Read the model definition and answer for the solid it produces. Units are mm, in the model's axes. Coordinates: 2 decimals unless noted, no trailing zeros.
Item 1: Determine the mould class of faces 1 (the face through (-276.225, 16, 0)), 2 (the face through (251, 7.27, -0.13)), 3 (the face through (-4, 16, -9.525)) for opening direction X: released by +X, released by -X, zero draft, split by the parting line, or undercut.
Item 2: Straight lines are drawn through the part: probe 1 along X at (y, z) = (21, -4.75) (3 decimals); probe 2 along X at (y, z) = (5.5, -4.75) (3 decimals); probe 3 along Y at (x, z) = (239, -6.5). For each, find the intervals that lie inside material, in ascending order.
Item 3: Each of these flat-tipped pins is pushed along its axis until it touches: P1, Ø2.5, axis at x = 225.23, y = 13.49, coming from the +Z side; P2, Ø7, axis at x = -260.55, y = 13.49, coming from the -Z side. Where does it stop, or does it pass through?
Item 4: Section A-A (z = 6.25) is taken. State how many separate pieces and enclosed holes the cut face has, then the cut area to 3 significant figures.
from build123d import *

# Parameters (mm, degrees)
SKETCH1_W                                         = 552.45
SKETCH1_H                                         = 19.05
BOSS_EXTRUDE1_DEPTH                               = 31.75
SKETCH2_R                                         = 10.2235
CUT_EXTRUDE1_DEPTH                                = 279.695560828
CSK_FOR_8_FLAT_HEAD_SOCKET_CAP_SCREW1_D           = 4.4958
CSK_FOR_8_FLAT_HEAD_SOCKET_CAP_SCREW1_CSINK_D     = 9.1186
CSK_FOR_8_FLAT_HEAD_SOCKET_CAP_SCREW1_CSINK_ANGLE = 82
CSK_FOR_8_FLAT_HEAD_MACHINE_SCREW1_D              = 4.4958
CSK_FOR_8_FLAT_HEAD_MACHINE_SCREW1_CSINK_D        = 8.4328
CSK_FOR_8_FLAT_HEAD_MACHINE_SCREW1_CSINK_ANGLE    = 82


with BuildPart() as part:
    # Sketch1 → Boss-Extrude1 (new body)
    with BuildSketch(Plane(origin=(0, 0, 0), x_dir=(1, 0, 0), z_dir=(0, 1, 0))):
        Rectangle(SKETCH1_W, SKETCH1_H)
    extrude(amount=BOSS_EXTRUDE1_DEPTH)

    # Sketch2 → Cut-Extrude1 (cut, through all)
    with BuildSketch(Plane(origin=(0, 0, -9.525), x_dir=(-1, 0, 0), z_dir=(0, 0, -1))):
        with Locations((-242.8875, 13.49375)):
            Circle(SKETCH2_R)
    extrude(amount=-CUT_EXTRUDE1_DEPTH, mode=Mode.SUBTRACT)

    # CSK for #8 Flat Head Socket Cap Screw1 (through all)
    with Locations(Plane(origin=(0, 0, -9.525), x_dir=(1, 0, 0), z_dir=(0, 0, -1))):
        with Locations((260.54685, -13.49375), (225.22815, -13.49375)):
            CounterSinkHole(CSK_FOR_8_FLAT_HEAD_SOCKET_CAP_SCREW1_D / 2, CSK_FOR_8_FLAT_HEAD_SOCKET_CAP_SCREW1_CSINK_D / 2, counter_sink_angle=CSK_FOR_8_FLAT_HEAD_SOCKET_CAP_SCREW1_CSINK_ANGLE)

    # CSK for #8 Flat Head Machine Screw1 (through all)
    with Locations(Plane(origin=(0, 0, -9.525), x_dir=(-1, 0, 0), z_dir=(0, 0, -1))):
        with Locations((260.54685, 13.49375)):
            CounterSinkHole(CSK_FOR_8_FLAT_HEAD_MACHINE_SCREW1_D / 2, CSK_FOR_8_FLAT_HEAD_MACHINE_SCREW1_CSINK_D / 2, counter_sink_angle=CSK_FOR_8_FLAT_HEAD_MACHINE_SCREW1_CSINK_ANGLE)


solid = part.part
Established:
1. face 1: released by -X
1. face 2: undercut
1. face 3: zero draft
2. probe 1: x = -276.225 to 235.947, 249.828 to 276.225
2. probe 2: x = -276.225 to 236.514, 249.261 to 276.225
2. probe 3: y = 0 to 4.04, 22.95 to 31.75
3. P1: passes through
3. P2: stops at z = -8.71
4. separate pieces: 1
4. enclosed holes: 4
4. area: 17,200 mm2
